The listing builds one solid part. Answer for the finished solid, in the listing's coordinates (mm). Face numbers are marked on the shaded views. A direction names the side the tool comes from. Give positions to 0.01 mm unless a question says otherwise; leave off trailing zeros. Order: outer loops, then holes, each group sorted by start corner. A loop starts at its lowest first (then second) coordinate and runs counter-clockwise, first axis right, second up. Notation, with made-up numbers: (57, 78) - (96, 78) arc R30 cw to (96, 109) - close; hole circle Ø7 at (7, 83.5). An arc over 180 degrees is marked (long way). Answer as a JSON object with one key per item and string values. Group by question number.
Q1. Consider line 1 (Y direction, x = 15.5, z = 28.5); line 2 (X direction, y = -40.5, z = 29). Determine where each line is inside the solid, lowest interval first.
Q2. A cutting plane is placed at A-A, the plane z = 22. Give the vertices of the cut face in (x, y).
Q3. For the marked faces 1, 2 and 3, determine the directions among +Z, -Z, +X, -X, +Y, -Y from which every point of the face is accessible in a straight line to the end or side of a thin tool.
Q4. A cutting plane is placed at B-B, the plane y = -17. Give the vertices of the cut face in (x, z).
Q5. Given pin 1 (3 mm diameter, centred on x = 21, y = -31.5, fed in from +Z); pin 2 (9.5 mm diameter, centred on y = -8.5, z = 21.5, fed in from +X); pin 3 (15 mm diameter, centred on x = 24.5, z = 20, fed in from -Y); pin 4 (4 mm diameter, centred on y = -22.5, z = 22.5, fed in from +X), each flat-ended and moving along its own axis, determine where each tip first touches the part or whether it passes through.
Q6. A cutting plane is placed at C-C, the plane x = 2. Give the vertices of the cut face in (y, z).
Q7. A cutting plane is placed at D-D, the plane y = -11.5. Give the vertices of the cut face in (x, z).
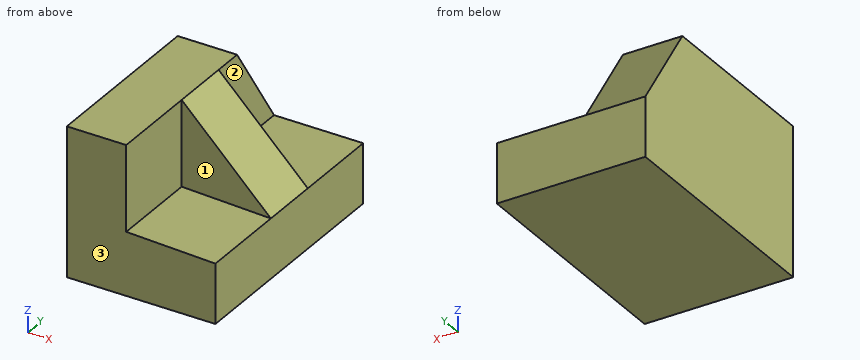
from build123d import *

# Parameters (mm, degrees)
F0_W     = 50.8
F0_H     = 31.75
F1_DEPTH = 31.75
F3_DEPTH = 31.751
F5_DEPTH = 19.05
F7_DEPTH = 31.751
F9_DEPTH = 19.05


with BuildPart() as f1:
    # F0 (on Right) → F1 (new body)
    with BuildSketch(Plane.YZ):
        with Locations((-25.4, 15.875)):
            Rectangle(F0_W, F0_H)
    extrude(amount=F1_DEPTH)

    # F2 (on face) → F3 (cut, through all)
    with BuildSketch(Plane.YZ.offset(31.75)):
        Polygon((0, 31.75), (-12.7, 31.75), (0, 12.7), align=None)
    extrude(amount=-F3_DEPTH, mode=Mode.SUBTRACT)

    # F4 (on face) → F5 (cut)
    with BuildSketch(Plane.YZ.offset(31.75)):
        Polygon((0, 12.7), (-12.7, 31.75), (-19.05, 31.75), (-19.05, 12.7), align=None)
    extrude(amount=-F5_DEPTH, mode=Mode.SUBTRACT)

    # F6 (on face) → F7 (cut, through all)
    with BuildSketch(Plane(origin=(0, -19.05, 0), x_dir=(-1, 0, 0), z_dir=(0, 1, 0))):
        Polygon((-31.75, 12.7), (-12.7, 31.75), (-31.75, 31.75), align=None)
    extrude(amount=-F7_DEPTH, mode=Mode.SUBTRACT)

    # F8 (on face) → F9 (cut)
    with BuildSketch(Plane.XZ.offset(50.8)):
        Polygon((31.75, 12.7), (12.7, 31.75), (12.7, 13.490058), align=None)
    extrude(amount=-F9_DEPTH, mode=Mode.SUBTRACT)


solid = f1.part
Reply:
{
 "1": {"line 1": "y = -31.75 to -19.05", "line 2": "x = 0 to 12.7"},
 "2": {"outline": "(0, -50.8) - (12.7, -50.8) - (12.7, -31.75) - (22.45, -31.75) - (22.45, -19.05) - (12.7, -19.05) - (12.7, -6.2) - (0, -6.2) - close"},
 "3": {"face 1": "+Z, +X, -Y", "face 2": "+Z, +X, +Y", "face 3": "+Z, -Z, +X, -X, -Y"},
 "4": {"outline": "(0, 0) - (31.75, 0) - (31.75, 12.7) - (12.7, 12.7) - (12.7, 31.75) - (0, 31.75) - close"},
 "5": {"pin 1": "stops at z = 24.95", "pin 2": "stops at x = 12.7", "pin 3": "stops at y = -50.8", "pin 4": "stops at x = 23.95"},
 "6": {"outline": "(-50.8, 0) - (0, 0) - (0, 12.7) - (-12.7, 31.75) - (-50.8, 31.75) - close"},
 "7": {"outline": "(0, 0) - (31.75, 0) - (31.75, 12.7) - (12.7, 12.7) - (12.7, 29.95) - (0, 29.95) - close"}
}
